For this review, take the finished solid that the model builds, in its own axes (mm). Coordinates: 2 decimals unless noted, no trailing zeros. Order: outer loops, then holes, each group sorted by start corner. A loop starts at its lowest first (then second) coordinate and runs counter-clockwise, first axis right, second up. Notation, with made-up numbers: M -35,-20 L -7,-20 A13 ccw -7,4 Z; hole C 56,19.25 d5. An arc over 180 degrees is marked long. Use CSV: the item, a comma, the result in double quotes.
```python
from build123d import *

# Parameters (mm, degrees)
SKETCH_1_W          = 66
SKETCH_1_H          = 40
EXTRUDE_1_DEPTH     = 3
SKETCH_2_R          = 1.575
SKETCH_2_R_2        = 4.1
SKETCH_2_R_3        = 2.1
SKETCH_2_W          = 10.2
SKETCH_2_H          = 20.2
CUT_EXTRUDE_1_DEPTH = 78.233412459
SKETCH_3_R          = 1
CUT_EXTRUDE_2_DEPTH = 78.233412459
FILLET_1_R          = 3


with BuildPart() as part:
    # 草图1 → 凸台-拉伸1 (new body)
    with BuildSketch(Plane.XY):
        with Locations((-33, -20)):
            Rectangle(SKETCH_1_W, SKETCH_1_H)
    extrude(amount=EXTRUDE_1_DEPTH)

    # 草图2 → 切除-拉伸1 (cut, through all)
    with BuildSketch(Plane.XY.offset(3)):
        with Locations((-61, -15)):
            Circle(SKETCH_2_R)
        with Locations(Location((-61, -25, 0), (0, 0, 180))):
            Circle(SKETCH_2_R)
        with Locations((-41, -25)):
            Circle(SKETCH_2_R)
        with Locations(Location((-41, -15, 0), (0, 0, 180))):
            Circle(SKETCH_2_R)
        with Locations((-15, -20)):
            Circle(SKETCH_2_R_2)
        with Locations((-24.25, -3.97853003)):
            Circle(SKETCH_2_R_3)
        with Locations((-5.75, -36.02146997)):
            Circle(SKETCH_2_R_3)
        with Locations((-51, -20)):
            Rectangle(SKETCH_2_W, SKETCH_2_H)
    extrude(amount=-CUT_EXTRUDE_1_DEPTH, mode=Mode.SUBTRACT)

    # 草图3 → 切除-拉伸2 (cut, through all)
    with BuildSketch(Plane.XY.offset(3)):
        with Locations((-45.9, -9.9)):
            Circle(SKETCH_3_R)
        with Locations((-45.9, -30.1)):
            Circle(SKETCH_3_R)
        with Locations((-56.1, -30.1)):
            Circle(SKETCH_3_R)
        with Locations((-56.1, -9.9)):
            Circle(SKETCH_3_R)
    extrude(amount=-CUT_EXTRUDE_2_DEPTH, mode=Mode.SUBTRACT)

    # 圆角1
    fillet_1_edges = [part.edges().sort_by_distance(p)[0] for p in [
        (0, -40, 1.5),
        (-66, -40, 1.5),
        (-66, 0, 1.5),
        (0, 0, 1.5),
    ]]
    fillet(fillet_1_edges, radius=FILLET_1_R)


solid = part.part
```
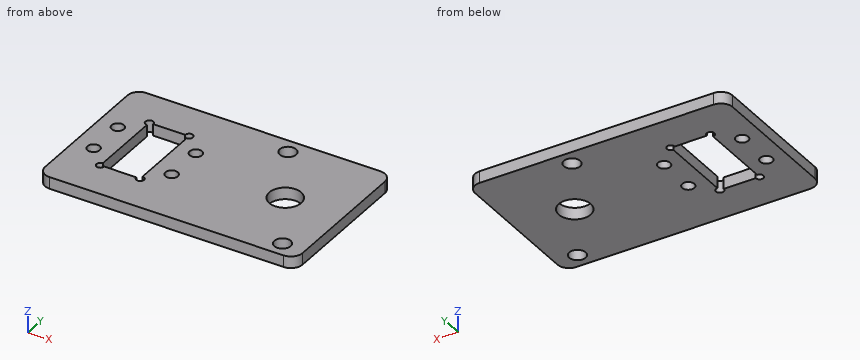
Item 1: Add section B-B on y = -25. State the section outline as (x, z) points (3 decimals), and give its area (4 significant figures).
Solutions:
outline,"M -66,0 L -62.575,0 L -62.575,3 L -66,3 Z; M -59.425,0 L -56.1,0 L -56.1,3 L -59.425,3 Z; M -45.9,0 L -42.575,0 L -42.575,3 L -45.9,3 Z; M -39.425,0 L 0,0 L 0,3 L -39.425,3 Z"
area,"148.5 mm^2"
Item 2: To check wall thickness, follow line 1 along Y through (x, z) = (-61, 0.7) (3 decimals); line 2 along X through (y, z) = (-23, 2); line 3 along Y through (x, z) = (-24.25, 1). State the ranges of each line that lie inside material, in increasing order. Write a range as [from, to].
Solutions:
line 1,"[-40, -26.575], [-23.425, -16.575], [-13.425, 0]"
line 2,"[-66, -56.1], [-45.9, -17.79], [-12.21, 0]"
line 3,"[-40, -6.08], [-1.88, 0]"
Item 3: Add section C-C on x = -15. State the section outline as (y, z) points.
Solutions:
outline,"M -40,0 L -24.1,0 L -24.1,3 L -40,3 Z; M -15.9,0 L 0,0 L 0,3 L -15.9,3 Z"
Item 4: Clearance check with a flat-ended pin moving along its axis: pin 1 Ø4 at (x, y) = (-41, -15) entering from -Z. State where the tip first meets the part, or that it passes through.
Solutions:
pin 1,"z = 0"
Item 5: Add section A-A on x = -61. State the section outline as (y, z) points (3 decimals), and give its area (3 significant figures).
Solutions:
outline,"M -40,0 L -26.575,0 L -26.575,3 L -40,3 Z; M -23.425,0 L -16.575,0 L -16.575,3 L -23.425,3 Z; M -13.425,0 L 0,0 L 0,3 L -13.425,3 Z"
area,"101 mm^2"
Item 6: Add section D-D on z = 1.35. State how many separate pieces and enclosed holes the cut face has, and give its area (3 significant figures).
Solutions:
separate pieces,"1"
enclosed holes,"8"
area,"2,310 mm^2"
